Here's how the part is built. I have some questions about the finished solid (model axes, mm). A direction names the side the tool comes from. Coordinates: 2 decimals unless noted, no trailing zeros. Write each loop counter-clockwise with the first axis right and the second up, starting at its lowest first coordinate (ties: lowest second). Pieces come first, ordered by that corner, then holes. Notation, with made-up numbers: M -7,69.25 L 22,69.25 A24 cw 22,86.25 Z; hole C 59,45 d1. An arc over 180 degrees is marked long. Write each question's results on one line, items separated by ' | '. Start each with the question number.
from build123d import *

# Parameters (mm, degrees)
SKETCH_1_W          = 450
SKETCH_1_H          = 63
EXTRUDE_1_DEPTH     = 20
CUT_EXTRUDE_START   = -20
SKETCH_2_W          = 445
SKETCH_2_H          = 55
CUT_EXTRUDE_1_DEPTH = 10
SKETCH_3_W          = 131.848612651
SKETCH_3_H          = 5
SKETCH_3_W_2        = 215.237788284
SKETCH_3_W_3        = 69.324505159
CUT_EXTRUDE_2_DEPTH = 64


with BuildPart() as part:
    # 草图1 → 凸台-拉伸1 (new body)
    with BuildSketch(Plane.XY):
        with Locations((-1046.220159151, 824.932360743)):
            Rectangle(SKETCH_1_W, SKETCH_1_H)
    extrude(amount=EXTRUDE_1_DEPTH)

    # 草图2 → 切除-拉伸1 (cut)
    with BuildSketch(Plane.XY.offset(20).offset(CUT_EXTRUDE_START)):
        with Locations((-1048.720159151, 824.932360743)):
            Rectangle(SKETCH_2_W, SKETCH_2_H)
    extrude(amount=CUT_EXTRUDE_1_DEPTH, mode=Mode.SUBTRACT)

    # 草图3 → 切除-拉伸2 (cut, through all)
    with BuildSketch(Plane.XZ.offset(-793.432360743)):
        with Locations((-1205.295852826, 2.5)):
            Rectangle(SKETCH_3_W, SKETCH_3_H)
        with Locations((-1014.979168507, 2.5)):
            Rectangle(SKETCH_3_W_2, SKETCH_3_H)
        with Locations((-855.882411731, 2.5)):
            Rectangle(SKETCH_3_W_3, SKETCH_3_H)
    extrude(amount=-CUT_EXTRUDE_2_DEPTH, mode=Mode.SUBTRACT)


solid = part.part
1) We'd pull the mould along Y, two halves only. Please class faces 1 (the flat face through (-825, 829, 5)), 2 (the flat face through (-1052, 797.432, 7)), 3 (the flat face through (-1049, 856.432, 12)): pulls with the +Y half, pulls with the -Y half, needs draft (parallel to the pull), parting line crosses it, or undercut.
2) For faces 4 (the flat face through (-1271.22, 824, 14)), 5 (the flat face through (-1052, 825, 10)), which set-ups out of +Z, -Z, +X, -X, +Y, -Y let a thin tool reach every point of the face, with its end or its side?
3) For pin 1 Ø2 at (y, z) = (855, 2) entering from -X; pin 2 Ø3 at (y, z) = (795, 2.5) entering from +X; pin 3 Ø8 at (y, z) = (817.5, 6.5) entering from -X; pin 4 Ø5.5 at (y, z) = (814.5, 7) entering from -X, each with a flat end and sliding along its axis, tell me the tip position at first contact or that it passes through.
4) I want a section at A-A, the plane x = -944.5. Write out the boundary of the cut face in (y, z).
5) I want a section at B-B, the plane y = 829. Write out the boundary of the cut face in (x, z).
6) Please list where these lines run through material, in increasing order: line 1 (Y direction, x = -906, z = 6.75); line 2 (Z direction, x = -991, y = 832); line 3 (X direction, y = 817, z = 6). Write a range as [from, to].
Output:
1) face 1: needs draft | face 2: undercut | face 3: pulls with the +Y half
2) face 4: +Z, -Z, -X, +Y, -Y | face 5: -Z, -X
3) pin 1: stops at x = -1139.37 | pin 2: stops at x = -890.54 | pin 3: stops at x = -1271.22 | pin 4: stops at x = -826.22
4) outline: M 793.43,5 L 797.43,5 L 797.43,10 L 852.43,10 L 852.43,5 L 856.43,5 L 856.43,20 L 793.43,20 Z
5) outline: M -1271.22,10 L -826.22,10 L -826.22,5 L -821.22,5 L -821.22,20 L -1271.22,20 Z
6) line 1: y = [793.43, 797.43], [852.43, 856.43] | line 2: z = [10, 20] | line 3: x = [-826.22, -821.22]
